```python
from build123d import *

# Parameters (mm, degrees)
F1_DEPTH = 15
F4_DEPTH = 1.25
F5_R     = 2.5
F6_DEPTH = 15
F8_DEPTH = 5


with BuildPart() as f1:
    # F0 (on Top) → F1 (new body)
    with BuildSketch(Plane.XY):
        with BuildLine():
            ThreePointArc((20, 41.3066352695), (5.8578643763, 35.4487708933), (0, 21.3066352695))
            Line((0, 21.3066352695), (0, -28.6933647305))
            Line((0, -28.6933647305), (10, -28.6933647305))
            Line((10, -28.6933647305), (10, 21.3066352695))
            ThreePointArc((10, 21.3066352695), (12.9289321881, 28.3777030814), (20, 31.3066352695))
            Line((20, 31.3066352695), (70, 31.3066352695))
            Line((70, 31.3066352695), (70, 41.3066352695))
            Line((70, 41.3066352695), (20, 41.3066352695))
        make_face()
    extrude(amount=F1_DEPTH)

    # F3 (on offset) → F4 (join, symmetric)
    with BuildSketch(Plane.XY.offset(7.5)):
        Polygon((10, 31.3066352695), (10, 16.3066352695), (25, 31.3066352695), align=None)
    extrude(amount=F4_DEPTH, both=True)

    # F5 (on face) → F6 (cut, through all)
    with BuildSketch(Plane.XY.offset(15)):
        with Locations((5, -13.6933647305)):
            Circle(F5_R)
        with Locations((5, -3.6933647305)):
            Circle(F5_R)
        with Locations((5, 6.3066352695)):
            Circle(F5_R)
        with Locations((30, 36.3066352695)):
            Circle(F5_R)
        with Locations((40, 36.3066352695)):
            Circle(F5_R)
    extrude(amount=-F6_DEPTH, mode=Mode.SUBTRACT)

    # F7 (on face) → F8 (join)
    with BuildSketch(Plane.XZ.offset(-31.3066352695)):
        with BuildLine():
            Line((70, 15), (47.0096189432, 15))
            ThreePointArc((47.0096189432, 15), (45, 7.5), (47.0096189432, 0))
            Line((47.0096189432, 0), (70, 0))
            Line((70, 0), (70, 15))
        make_face()
        with BuildLine():
            ThreePointArc((47.0096189432, 0), (63.8822856765, -6.9888873943), (75, 7.5))
            ThreePointArc((75, 7.5), (63.8822856765, 21.9888873943), (47.0096189432, 15))
            Line((47.0096189432, 15), (70, 15))
            Line((70, 15), (70, 0))
            Line((70, 0), (47.0096189432, 0))
        make_face()
    extrude(amount=-F8_DEPTH)


solid = f1.part
```
CAD build for the part. Positions are in the model's coordinates, mm. A direction names the side the tool comes from. Coordinates: 2 decimals unless noted, no trailing zeros. Write each loop counter-clockwise with the first axis right and the second up, starting at its lowest first coordinate (ties: lowest second). Pieces come first, ordered by that corner, then holes.
(1) Flat gauge pins, fed straight in: pin 1 (6 mm diameter, centred on x = 5, y = 6.31, fed in from +Z); pin 2 (4.5 mm diameter, centred on x = 20.5, y = 27, fed in from -Z); pin 3 (12 mm diameter, centred on x = 28, z = -3, fed in from -Y). Where does each tip first touch, or does it go through?
(2) Cut at A-A, the plane x = 30. List the corners of the cut face in (y, z), and give its area (3 significant figures).
(3) Drill centre lines: probe 1 along Y at (x, z) = (5, 12.25); probe 2 along Y at (x, z) = (30, 9.75); probe 3 along Y at (x, z) = (67, 8). Where is each one in solid material? Low to high.
(4) Cut at D-D, the plane y = 29. List the corners of the cut face in (x, z).
(5) Cut at B-B, the plane z = 11.5. List the corners of the cut face in (x, y).
(6) 3-axis set-ups, long thin cutter, end or side, ignore diameter. For faces 5 (the face through (0, -3, 7)), 6 (the face through (17.395, 23.702, 7.518)), 7 (the face through (16, 26, 6.25)), 8 (the face through (16, 26, 8.75)), 9 (the face through (70, 39, 7)): which of +Z, -Z, +X, -X, +Y, -Y reach the whole face in a straight line?
(7) Two-plate mould, pull along Y, no slides. Class faces 1 (the face through (12.85, 28.3, 11.83)), 2 (the face through (9, 17, 0)), 3 (the face through (45, 41.307, 7)), 4 (the face through (7.31, -4.65, 7.6)): +Y half, -Y half, draft (parallel to the pull), parting line (faces both ways), or undercut.
(8) Cut at C-C, the plane x = 5. List the corners of the cut face in (y, z).
Geometry says:
1. pin 1: stops at z = 15
1. pin 2: stops at z = 6.25
1. pin 3: stops at y = 31.31
2. outline: (31.31, 0) - (33.81, 0) - (33.81, 15) - (31.31, 15) - close; (38.81, 0) - (41.31, 0) - (41.31, 15) - (38.81, 15) - close
2. area: 75.0 mm2
3. probe 1: y = -28.69 to -16.19, -11.19 to -6.19, -1.19 to 3.81, 8.81 to 34.54
3. probe 2: y = 31.31 to 33.81, 38.81 to 41.31
3. probe 3: y = 31.31 to 41.31
4. outline: (1.54, 0) - (13.61, 0) - (13.61, 6.25) - (22.69, 6.25) - (22.69, 8.75) - (13.61, 8.75) - (13.61, 15) - (1.54, 15) - close
5. outline: (0, -28.69) - (10, -28.69) - (10, 21.31) arc R10 cw to (20, 31.31) - (74.46, 31.31) - (74.46, 36.31) - (70, 36.31) - (70, 41.31) - (20, 41.31) arc R20 ccw to (0, 21.31) - close; hole circle Ø5 at (5, -13.69); hole circle Ø5 at (5, -3.69); hole circle Ø5 at (5, 6.31); hole circle Ø5 at (30, 36.31); hole circle Ø5 at (40, 36.31)
6. face 5: +Z, -Z, -X, +Y, -Y
6. face 6: +Z, -Z, +X, -Y
6. face 7: -Z, +X, -Y
6. face 8: +Z, +X, -Y
6. face 9: +Z, -Z, +X, +Y
7. face 1: -Y half
7. face 2: draft
7. face 3: +Y half
7. face 4: undercut
8. outline: (-28.69, 0) - (-16.19, 0) - (-16.19, 15) - (-28.69, 15) - close; (-11.19, 0) - (-6.19, 0) - (-6.19, 15) - (-11.19, 15) - close; (-1.19, 0) - (3.81, 0) - (3.81, 15) - (-1.19, 15) - close; (8.81, 0) - (34.54, 0) - (34.54, 15) - (8.81, 15) - close
